Here's how the part is built. I have some questions about the finished solid (model axes, mm). Face numbers are marked on the shaded views. A direction names the side the tool comes from. Round coordinates to 2 decimals unless told otherwise and drop trailing zeros. Loops run counter-clockwise (first coordinate to the right, second up) from the corner with the lowest first, then second, coordinate; pieces in that order, holes last. Notation, with made-up numbers: M 50.25,16 L 99.25,16 A16 ccw 99.25,37 Z; hole C 45,12.25 d9. An arc over 180 degrees is marked long. Answer as a JSON object with one key per item and string values.
Autodesk Inventor part; units mm, degrees
ref_plane "Work Plane1" through (0, 0, 3) normal (0, 0, 1) x (1, 0, 0)
ref_plane "YZ Plane" through (0, 0, 0) normal (1, 0, 0) x (0, 1, 0)
ref_plane "XZ Plane" through (0, 0, 0) normal (0, 1, 0) x (-1, 0, 0)
sketch "Sketch1" plane through (0, 0, 0) normal (0, 0, 1) x (1, 0, 0)
  circle A0 centre (0, 0) radius 7.5
  circle A1 centre (0, 0) radius 3
  dimension "d0" = 15
  dimension "d1" = 6
extrude "Extrusion1" add sketch "Sketch1" along normal blind 10
ref_plane "Work Plane1" through (0, 0, 3) normal (0, 0, 1) x (1, 0, 0)
sketch "Sketch2" plane through (0, 0, 3) normal (0, 0, 1) x (1, 0, 0)
  line L0 (-5.5, -2.6) -> (-3.3, -2.6)
  line L1 (-3.3, -2.6) -> (-3.3, 2.6)
  line L2 (-3.3, 2.6) -> (-5.5, 2.6)
  line L3 (-5.5, 2.6) -> (-5.5, -2.6)
  point P0 (0, 0)
  point P1 (-5.5, 0)
  dimension "d5" = 5.5
  dimension "d6" = 2.2
  dimension "d7" = 5.2
extrude "Extrusion2" cut sketch "Sketch2" along normal blind 7
sketch "Sketch4" plane through (0, 0, 0) normal (1, 0, 0) x (0, 1, 0)
  circle A0 centre (0, 7) radius 1.5
  line L0 (-2.1, 0) -> (2.1, 0)
  point P0 (0, 0)
  dimension "d12" = 3
  dimension "d13" = 7
extrude "Extrusion3" cut sketch "Sketch4" against normal blind 8
sketch "Sketch5" plane through (0, 0, 0) normal (0, 1, 0) x (-1, 0, 0)
  line L0 (7.5, 0) -> (7.5, 10)
  line L1 (7.5, 4) -> (7, 4)
  line L2 (7, 4) -> (7, 10)
  line L3 (7, 10) -> (7.5, 10)
  line L4 (7.5, 10) -> (7.5, 4)
  line L5 (-1.5, 0) -> (9, 0)
  point P0 (0, 0)
  dimension "d16" = 6
  dimension "d17" = 10
  dimension "d18" = 0.5
extrude "Extrusion4" cut sketch "Sketch5" along normal mid plane 8
sketch "Sketch6" plane through (0, 0, 0) normal (0, 0, -1) x (-1, 0, 0)
  point P0 (0, 0)
properties part number "Acople eje motor"
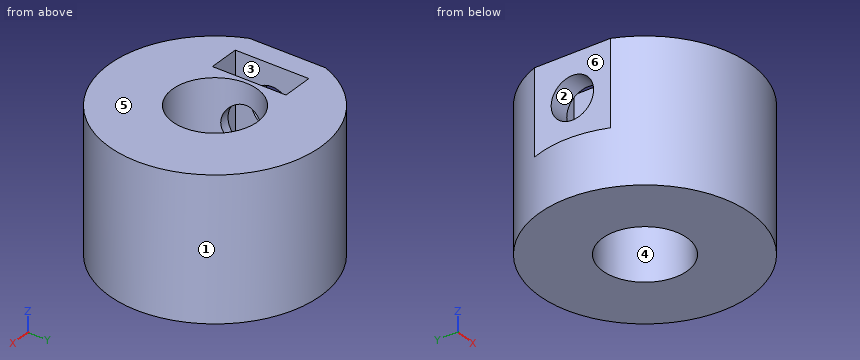
Item 1: I want a section at B-B on y = 0. List the corners of the cut face in (x, z) for me.
Solution:
{"outline": "M -7.5,0 L -3,0 L -3,5.5 L -3.3,5.5 L -3.3,3 L -5.5,3 L -5.5,5.5 L -7,5.5 L -7,4 L -7.5,4 Z; M -7,8.5 L -5.5,8.5 L -5.5,10 L -7,10 Z; M -3.3,8.5 L -3,8.5 L -3,10 L -3.3,10 Z; M 3,0 L 7.5,0 L 7.5,10 L 3,10 Z"}
Item 2: We'd pull the mould along X, two halves only. Please class the marked faces 4, 5 and 6: +X half, -X half, draft (parallel to the pull), parting line (faces both ways), or undercut.
Solution:
{"face 4": "undercut", "face 5": "draft", "face 6": "-X half"}
Item 3: I want a section at D-D on z = 7. List the corners of the cut face in (x, y) for me.
Solution:
{"outline": "M -7,-2.69 A7.5 ccw long -7,2.69 L -7,1.5 L -5.5,1.5 L -5.5,2.6 L -3.3,2.6 L -3.3,1.5 L -2.6,1.5 A3 cw long -2.6,-1.5 L -3.3,-1.5 L -3.3,-2.6 L -5.5,-2.6 L -5.5,-1.5 L -7,-1.5 Z"}
Item 4: I want a section at C-C on z = 3.5. List the corners of the cut face in (x, y) for me, plus the area to 3 significant figures.
Solution:
{"outline": "C 0,0 d15; hole M -5.5,-2.6 L -3.3,-2.6 L -3.3,2.6 L -5.5,2.6 Z; hole C 0,0 d6", "area": "137 mm2"}
Item 5: For the marked faces 1, 2 and 3, which set-ups out of +Z, -Z, +X, -X, +Y, -Y let a thin tool reach every point of the face, with its end or its side?
Solution:
{"face 1": "+Z, -Z", "face 2": "-X", "face 3": "+Z"}
Item 6: If I drill on L1, parallel to X at y = 0, z = 3.5; L2, parallel to Y at x = 0.25, z = 6.25; L3, parallel to Y at x = -3.1, z = 7, over which ranges is the centre line in solid material (lowest first)? Write a range as from..to.
Solution:
{"L1": "x = -7.5..-5.5, -3.3..-3, 3..7.5", "L2": "y = -7.5..-2.99, 2.99..7.5", "L3": "y = -6.83..-1.5, 1.5..6.83"}
Item 7: I want a section at A-A on x = 0. List the corners of the cut face in (y, z) for me.
Solution:
{"outline": "M -7.5,0 L -3,0 L -3,10 L -7.5,10 Z; M 3,0 L 7.5,0 L 7.5,10 L 3,10 Z"}
Item 8: For P1, Ø1.1, axis at x = -4.5, y = -0.5, coming from the +Z side; P2, Ø1.6, axis at y = 0.5, z = 7, coming from the -X side; P3, Ø1.8, axis at x = -4, z = 6.5, coming from the -Y side, each with a flat end and sliding along its axis, tell me the tip position at first contact or that it passes through.
Solution:
{"P1": "stops at z = 3", "P2": "stops at x = 2.7", "P3": "stops at y = -6.83"}
